```python
from build123d import *

# Parameters (mm, degrees)
BOSS_EXTRUDE1_DEPTH = 4.875
SKETCH3_OUTSIDE_W   = 32.934
SKETCH3_OUTSIDE_H   = 113.184
SKETCH3_OUTSIDE_R   = 4.9
CUT_EXTRUDE1_DEPTH  = 14.716884
SKETCH4_R           = 3.75
CUT_EXTRUDE2_DEPTH  = 9.75


with BuildPart() as part:
    # Sketch2 → Boss-Extrude1 (new body, symmetric)
    with BuildSketch(Plane(origin=(0, 0, 0), x_dir=(0, 0, -1), z_dir=(1, 0, 0))):
        with BuildLine():
            Line((0, -0.695639294), (0, 0.695639294))
            ThreePointArc((0, 0.695639294), (-0.743104239, 7.331455024), (-2.93560336, 13.638530568))
            Line((-2.93560336, 13.638530568), (-14.510732773, 37.842851454))
            ThreePointArc((-14.510732773, 37.842851454), (-12.494794947, 44.333127989), (-5.869704015, 42.817916797))
            Line((-5.869704015, 42.817916797), (17.022523842, 9.264166407))
            ThreePointArc((17.022523842, 9.264166407), (20.611838468, 6.058101563), (25.283115813, 4.9))
            Line((25.283115813, 4.9), (40, 4.9))
            Line((40, 4.9), (40, -4.9))
            Line((40, -4.9), (25.283115813, -4.9))
            ThreePointArc((25.283115813, -4.9), (20.611838468, -6.058101563), (17.022523842, -9.264166407))
            Line((17.022523842, -9.264166407), (-5.869704015, -42.817916797))
            ThreePointArc((-5.869704015, -42.817916797), (-12.494794947, -44.333127989), (-14.510732773, -37.842851454))
            Line((-14.510732773, -37.842851454), (-2.93560336, -13.638530568))
            ThreePointArc((-2.93560336, -13.638530568), (-0.743104239, -7.331455024), (0, -0.695639294))
        make_face()
    extrude(amount=BOSS_EXTRUDE1_DEPTH, both=True)

    # Sketch3 outside → Cut-Extrude1 (cut)
    with BuildSketch(Plane(origin=(0, 0, -40), x_dir=(-1, 0, 0), z_dir=(0, 0, -1))):
        Rectangle(SKETCH3_OUTSIDE_W, SKETCH3_OUTSIDE_H)
        Circle(SKETCH3_OUTSIDE_R, mode=Mode.SUBTRACT)
    extrude(amount=-CUT_EXTRUDE1_DEPTH, mode=Mode.SUBTRACT)

    # Sketch4 → Cut-Extrude2 (cut)
    with BuildSketch(Plane(origin=(4.875, 0, 0), x_dir=(0, 0, -1), z_dir=(1, 0, 0))):
        with Locations((-7.144836337, 35.884581199)):
            Circle(SKETCH4_R)
        with Locations((-7.144836337, -35.884581199)):
            Circle(SKETCH4_R)
    extrude(amount=-CUT_EXTRUDE2_DEPTH, mode=Mode.SUBTRACT)


solid = part.part
```
Design review of the part built by this model. Coordinates are the model's own, in mm. A direction names the side the tool comes from. Give positions to 0.01 mm unless a question says otherwise; leave off trailing zeros. Write each loop counter-clockwise with the first axis right and the second up, starting at its lowest first coordinate (ties: lowest second). Pieces come first, ordered by that corner, then holes. Notation, with made-up numbers: (49.5, 79) - (71.5, 79) arc R22 ccw to (71.5, 91) - close; hole circle Ø6 at (69.25, 75.25). An arc over 180 degrees is marked (long way). Return JSON: item names as keys, results as strings. Group by question number.
(1) We need section C-C, the plane y = -33. Give the boundary of the cut face in (x, z) (3 decimals).
(2) Mouldability with a two-part tool opening along Z and no side actions: class faces 5 (the cylindrical face through (0.068, -32.166, 7.633)), 6 (the flat face through (4.875, 4, -4)), 7 (the cylindrical face through (0.068, -6.027, -20.672)), 8 (the cylindrical face through (0.068, 32.224, 7.958)) as +Z half, -Z half, draft (parallel to the pull), parting line (faces both ways), or undercut.
(3) We need section A-A, the plane z = 1.5. Give the boundary of the cut face in (x, y) (3 decimals).
(4) To check wall thickness, follow probe 1 along Y at (x, z) = (1, 6); probe 2 along Z at (x, y) = (-1.5, -36); probe 3 along Y at (x, z) = (-0.75, 8). State the ranges of each line that lie inside material, in increasing order.
(5) Machinability: for faces 1 (the cylindrical face through (0.068, -7.423, 0.764)), 2 (the cylindrical face through (0.1, -4.9, -32.7)), 3 (the flat face through (-4, 4, -25.283)), 4 (the flat face through (4, -4, -25.283)), which of the approach directions +Z, -Z, +X, -X, +Y, -Y give a long, thin tool a straight path to every point of the face, cutting with its end or side? Answer none if there is none.
(6) We need section B-B, the plane x = 2.75. Give the boundary of the cut face in (y, z), then the cut area to 3 significant figures.
(7) Insertion check: pin 1 (1 mm diameter, centred on x = -1, y = 14, fed in from +Z); pin 2 (1 mm diameter, centred on x = -0.5, y = -18, fed in from -Z); pin 3 (5 mm diameter, centred on x = -0.5, z = -13.5, fed in from -Y). Each pin has a flat end and moves straight along its axis. Give the tip position at first contact, or say it passes through.
(8) We need section D-D, the plane z = 10. Give the boundary of the cut face in (x, y) (3 decimals), then the cut area to 3 significant figures.
Reported:
{
 "1": {"outline": "(-4.875, -0.829) - (4.875, -0.829) - (4.875, 4.749) - (-4.875, 4.749) - close; (-4.875, 9.541) - (4.875, 9.541) - (4.875, 12.195) - (-4.875, 12.195) - close"},
 "2": {"face 5": "undercut", "face 6": "draft", "face 7": "-Z half", "face 8": "undercut"},
 "3": {"outline": "(-4.875, -36.413) - (4.875, -36.413) - (4.875, -10.063) - (-4.875, -10.063) - close; (-4.875, 10.063) - (4.875, 10.063) - (4.875, 36.413) - (-4.875, 36.413) - close"},
 "4": {"probe 1": "y = -43 to -39.46, -32.31 to -20.05, 20.05 to 32.31, 39.46 to 43", "probe 2": "z = 1.22 to 3.4, 10.89 to 13.63", "probe 3": "y = -44.58 to -39.54, -32.23 to -24.23, 24.23 to 32.23, 39.54 to 44.58"},
 "5": {"face 1": "+Z, +X, -X", "face 2": "-Z, -Y", "face 3": "-Z, -X, +Y", "face 4": "-Z, +X, -Y"},
 "6": {"outline": "(-42.82, 5.87) - (-9.26, -17.02) arc R10 cw to (-4.9, -25.28) - (-4.06, -25.28) - (-4.06, -40) - (4.06, -40) - (4.06, -25.28) - (4.9, -25.28) arc R10 cw to (9.26, -17.02) - (42.82, 5.87) arc R5 ccw to (37.84, 14.51) - (13.64, 2.94) arc R30 cw to (0.7, 0) - (-0.7, 0) arc R30 cw to (-13.64, 2.94) - (-37.84, 14.51) arc R5 ccw to start; hole circle Ø7.5 at (-35.88, 7.14); hole circle Ø7.5 at (35.88, 7.14)", "area": "1,440 mm2"},
 "7": {"pin 1": "stops at z = 3.35", "pin 2": "stops at z = -11.4", "pin 3": "stops at y = -18.09"},
 "8": {"outline": "(-4.875, -45) - (4.875, -45) - (4.875, -38.316) - (-4.875, -38.316) - close; (-4.875, -33.453) - (4.875, -33.453) - (4.875, -28.411) - (-4.875, -28.411) - close; (-4.875, 28.411) - (4.875, 28.411) - (4.875, 33.453) - (-4.875, 33.453) - close; (-4.875, 38.316) - (4.875, 38.316) - (4.875, 45) - (-4.875, 45) - close", "area": "229 mm2"}
}
